Geometry: final body of the model. Coordinates: model frame, mm. Give positions to 0.01 mm unless a question says otherwise; leave off trailing zeros. Loops run counter-clockwise (first coordinate to the right, second up) from the corner with the lowest first, then second, coordinate; pieces in that order, holes last.
1. Material intervals for line 1 along Y through (x, z) = (0, 23); line 2 along X through (y, z) = (0.5, 591); line 3 along Y through (x, z) = (0.75, 465), sorted ascending.
2. Section B-B, the plane y = -5.5. Output: boundary loops of the cut face in (x, z).
3. Section C-C, the plane x = -5.25. Output: boundary loops of the cut face in (y, z).
4. Section A-A, the plane z = 127.5. Output: boundary loops of the cut face in (x, y), then the cut area to 3 significant figures.
5. First-contact query: P1, Ø1, axis at x = 1, z = 552, coming from the -Y side; P2, Ø6, axis at y = -6, z = 809, coming from the +X side; P3, Ø4.5, axis at x = 0, y = 0, coming from the +Z side. Flat tips, straight axial feed; report the tip coordinate or a pass-through.
Autodesk Inventor part; units mm, degrees
ref_plane "YZ Plane" through (0, 0, 0) normal (1, 0, 0) x (0, 1, 0)
ref_plane "XZ Plane" through (0, 0, 0) normal (0, 1, 0) x (-1, 0, 0)
ref_plane "XY Plane" through (0, 0, 0) normal (0, 0, 1) x (1, 0, 0)
sketch "Szkic1" plane through (0, 0, 0) normal (0, 0, 1) x (1, 0, 0)
  circle A0 centre (0, 0) radius 8
  line L0 (0, 8) -> (0, 0) construction
  dimension "d0" = 16
extrude "Wyciągnięcie proste1" add sketch "Szkic1" along normal blind 1000
sketch "Szkic2" plane through (0, 0, 1000) normal (0, 0, 1) x (1, 0, 0)
  circle A0 centre (0, 0) radius 8
  line L0 (0, 8) -> (0, -8)
  line L1 (-8, 0) -> (8, 0)
hole "Otwór1" at (0, 0, 1000) direction (0, 0, -1) diameter 4.9784 depth 32 tip angle 118
sketch "Szkic3" plane through (0, 0, 0) normal (0, 0, -1) x (-1, 0, 0)
  circle A0 centre (0, 0) radius 8
  line L0 (0, 8) -> (0, -8)
  line L1 (-8, 0) -> (8, 0)
hole "Otwór2" at (0, 0, 0) direction (0, 0, 1) diameter 4.9784 depth 32 tip angle 118
properties part number "walek_liniowy_fi16_L1000"
Answers below:
1. line 1: y = -8 to -2.49, 2.49 to 8
1. line 2: x = -7.98 to 7.98
1. line 3: y = -7.96 to 7.96
2. outline: (-5.81, 0) - (5.81, 0) - (5.81, 1000) - (-5.81, 1000) - close
3. outline: (-6.04, 0) - (6.04, 0) - (6.04, 1000) - (-6.04, 1000) - close
4. outline: circle Ø16 at (0, 0)
4. area: 201 mm2
5. P1: stops at y = -7.98
5. P2: stops at x = 7.42
5. P3: stops at z = 967.86
